from build123d import *

# Parameters (mm, degrees)
BOSS_EXTRUDE1_DEPTH = 3
BOSS_EXTRUDE2_DEPTH = 4


with BuildPart() as part:
    # Sketch1 → Boss-Extrude1 (new body)
    with BuildSketch(Plane(origin=(0, 0, 0), x_dir=(1, 0, 0), z_dir=(0, 1, 0))):
        Polygon((0, 0), (-2, 4), (0, 4), align=None)
    extrude(amount=BOSS_EXTRUDE1_DEPTH)

    # Sketch2 → Boss-Extrude2 (add)
    with BuildSketch(Plane(origin=(0, 0, -4), x_dir=(-1, 0, 0), z_dir=(0, 0, -1))):
        Polygon((0, 3), (-2, 5), (-2, 3), (-4, 0), (0, 0), align=None)
    extrude(amount=-BOSS_EXTRUDE2_DEPTH)


solid = part.part
Verification items for the finished model (mm, model axes). A direction names the side the tool comes from. Coordinates: 2 decimals unless noted, no trailing zeros. Order: outer loops, then holes, each group sorted by start corner. A loop starts at its lowest first (then second) coordinate and runs counter-clockwise, first axis right, second up. Notation, with made-up numbers: (-19.5, 55) -> (30.5, 55) arc R28 ccw to (30.5, 93) -> close; hole circle Ø7 at (86.5, 53.25). An arc over 180 degrees is marked (long way). Use CSV: the item, a comma, the result in double quotes. Start each with the question number.
Q1. Depth check by flat-ended pin: P1, Ø3, axis at x = -1, y = 2.5, coming from the +Z side; P2, Ø0.6, axis at x = -1, z = -3, coming from the +Y side; P3, Ø1.5, axis at y = 4.5, z = -2.5, coming from the +X side. Enter the tip coordinate at first touch or a pass-through.
Q2. Thickness scan on line 1 along Y through (x, z) = (-0.7, -3.2); line 2 along Z through (x, y) = (-0.2, 2.45); line 3 along Y through (x, z) = (1.55, -2.7). Record the ranges inside material, lowest first.
Q3. Section check C-C, the plane x = 1.5. Record the cut outline in (y, z).
Q4. Section check A-A, the plane z = -3.6. Record the cut outline in (x, y).
Q5. Tool access check on faces 1 (the flat face through (2, 4, -2)), 2 (the flat face through (-0.8, 3, -2.5)), 3 (the flat face through (2, 0, -2)). Record the directions out of +Z, -Z, +X, -X, +Y, -Y that give a thin tool (end or side, any length) a straight path to the whole face; none if there is none.
Q6. Section check D-D, the plane z = -2.7. Record the cut outline in (x, y).
Q7. Section check B-B, the plane y = 0.3. Record the cut outline in (x, z), and give its area (3 significant figures).
Returned:
1,P1,"stops at z = 0"
1,P2,"stops at y = 3"
1,P3,"stops at x = 2"
2,line 1,"y = 0 to 3"
2,line 2,"z = -4 to -0.4"
2,line 3,"y = 0 to 4.55"
3,outline,"(0, -4) -> (4.5, -4) -> (4.5, 0) -> (0, 0) -> close"
4,outline,"(-1.8, 0) -> (4, 0) -> (2, 3) -> (2, 5) -> (0, 3) -> (-1.8, 3) -> close"
5,face 1,"+Z, -Z, +X, +Y"
5,face 2,"+Z, -Z, -X, +Y"
5,face 3,"+Z, -Z, +X, -X, -Y"
6,outline,"(-1.35, 0) -> (4, 0) -> (2, 3) -> (2, 5) -> (0, 3) -> (-1.35, 3) -> close"
7,outline,"(-2, -4) -> (3.8, -4) -> (3.8, 0) -> (0, 0) -> close"
7,area,"19.2 mm^2"
